Source: CAD feature listing. Evaluate the final solid. Frame: model axes, mm. Face numbers are marked on the shaded views. Give positions to 0.01 mm unless a question says otherwise; leave off trailing zeros. Order: outer loops, then holes, each group sorted by start corner. A loop starts at its lowest first (then second) coordinate and runs counter-clockwise, first axis right, second up. Notation, with made-up numbers: (73.5, -27.75) - (120.5, -27.75) arc R36 cw to (120.5, 11.25) - close; hole circle Ø9 at (-24, 35). An arc over 180 degrees is marked (long way). Use CSV: the item, a comma, the result in double quotes.
```python
from build123d import *

# Parameters (mm, degrees)
SKETCH1_R             = 18
BOSS_EXTRUDE1_DEPTH   = 4.7625
M8_CLEARANCE_HOLE1_D  = 9
M6X1_0_TAPPED_HOLE1_D = 5
CHAMFER1_SIZE         = 1


with BuildPart() as part:
    # Sketch1 → Boss-Extrude1 (new, symmetric)
    with BuildSketch(Plane.XY):
        Polygon((-30, -23.5), (24.784271247, -23.5), (70, 21.715728753), (70, 107.5), (-30, 107.5), align=None)
        with Locations(Location((0, 0, 0), (0, 0, 180))):
            Circle(SKETCH1_R, mode=Mode.SUBTRACT)
    extrude(amount=BOSS_EXTRUDE1_DEPTH, both=True)

    # M8 Clearance Hole1 (through all)
    with Locations(Plane.XY.offset(4.7625)):
        with Locations((-20, 90), (15, 90), (50, 90), (50, 60), (50, 30)):
            Hole(M8_CLEARANCE_HOLE1_D / 2)

    # M6x1.0 Tapped Hole1 (through all)
    with Locations(Plane.XY.offset(4.7625)):
        with Locations((16.617009358, 16.617009358), (23.5, 0), (16.617009358, -16.617009358), (-16.617009358, -16.617009358), (-23.5, 0), (-16.617009358, 16.617009358)):
            Hole(M6X1_0_TAPPED_HOLE1_D / 2)

    # Chamfer1
    chamfer1_edges = [part.edges().sort_by_distance(p)[0] for p in [
        (-30, 107.5, 0),
        (70, 107.5, 0),
        (-30, -23.5, 0),
    ]]
    chamfer(chamfer1_edges, length=CHAMFER1_SIZE)


solid = part.part
```
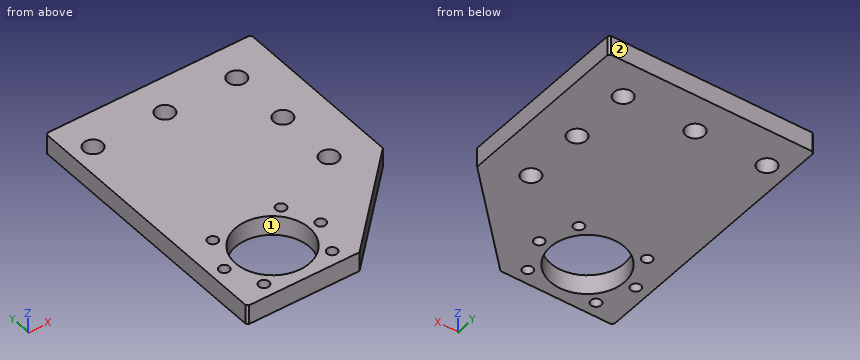
Item 1: Section A-A on y = 90. Return the cut outline in (x, z).
Filled in:
outline,"(-30, -4.76) - (-24.5, -4.76) - (-24.5, 4.76) - (-30, 4.76) - close; (-15.5, -4.76) - (10.5, -4.76) - (10.5, 4.76) - (-15.5, 4.76) - close; (19.5, -4.76) - (45.5, -4.76) - (45.5, 4.76) - (19.5, 4.76) - close; (54.5, -4.76) - (70, -4.76) - (70, 4.76) - (54.5, 4.76) - close"
Item 2: Mould query, pull axis X, two halves, no side actions, for the marked faces 1 and 2. Classes: released by +X, released by -X, zero draft, split by the parting line, or undercut.
Filled in:
face 1,"undercut"
face 2,"zero draft"
Item 3: Section C-C on y = -10. Return the cut outline in (x, z), then the cut area to 3 significant figures.
Filled in:
outline,"(-30, -4.76) - (-14.97, -4.76) - (-14.97, 4.76) - (-30, 4.76) - close; (14.97, -4.76) - (38.28, -4.76) - (38.28, 4.76) - (14.97, 4.76) - close"
area,"365 mm2"
Item 4: Section B-B on x = 0. Return the cut outline in (y, z).
Filled in:
outline,"(-23.5, -4.76) - (-18, -4.76) - (-18, 4.76) - (-23.5, 4.76) - close; (18, -4.76) - (107.5, -4.76) - (107.5, 4.76) - (18, 4.76) - close"
Item 5: First-contact query: pin 1 (2 mm diameter, centred on x = 57, y = 6, fed in from -Z); pin 2 (1 mm diameter, centred on x = 53, z = -3.5, fed in from -Y). Flat tips, straight axial feed; report the tip coordinate or a pass-through.
Filled in:
pin 1,"passes through"
pin 2,"stops at y = 4.22"
Item 6: Material intervals for line 1 (Y direction, x = -20, z = -0.25); line 2 (X direction, y = 15.5, z = -0.5); line 3 (Y direction, x = 13, z = 4), sorted ascending. Write a range as from..to.
Filled in:
line 1,"y = -23.5..85.5, 94.5..107.5"
line 2,"x = -30..-18.85, -14.38..-9.15, 9.15..14.38, 18.85..63.78"
line 3,"y = -23.5..-12.45, 12.45..85.97, 94.03..107.5"
Item 7: Section D-D on x = 50. Return the cut outline in (y, z).
Filled in:
outline,"(1.72, -4.76) - (25.5, -4.76) - (25.5, 4.76) - (1.72, 4.76) - close; (34.5, -4.76) - (55.5, -4.76) - (55.5, 4.76) - (34.5, 4.76) - close; (64.5, -4.76) - (85.5, -4.76) - (85.5, 4.76) - (64.5, 4.76) - close; (94.5, -4.76) - (107.5, -4.76) - (107.5, 4.76) - (94.5, 4.76) - close"
